Work out the finished part from the listing and answer in its coordinate system (mm). A direction names the side the tool comes from. Give positions to 0.01 mm unless a question says otherwise; leave off trailing zeros. Write each loop counter-clockwise with the first axis right and the second up, starting at its lowest first coordinate (ties: lowest second). Pieces come first, ordered by that corner, then holes. Notation, with made-up numbers: (-21, 62) - (-11, 62) arc R16 cw to (-11, 77) - close; hole circle Ø10 at (80, -23.5). An arc over 180 degrees is marked (long way). Write item = value, one per line.
from build123d import *

# Parameters (mm, degrees)
SKETCH3_R   = 12.7
SKETCH3_R_2 = 8.73125


with BuildPart() as part:
    # Sweep1: sweep along a path in Sketch1
    with BuildLine(Plane.XY) as sweep1_path:
        Line((0, 0), (0, 241.3))
        Line((0, 241.3), (736.6, 241.3))
        Line((736.6, 241.3), (736.6, 0))
    # Sketch3 → Sweep1 (sweep)
    with BuildSketch(Plane(origin=(0, 0, 0), x_dir=(1, 0, 0), z_dir=(0, 1, 0))):
        Circle(SKETCH3_R)
        Circle(SKETCH3_R_2, mode=Mode.SUBTRACT)
    sweep(path=sweep1_path.line, transition=Transition.RIGHT)


solid = part.part
1. Find section D-D, the plane y = 241.3. Give the vertices of the cut face in (x, z).
Solution:
outline = (0, -12.7) - (736.6, -12.7) arc R12.7 ccw to (736.6, 12.7) - (0, 12.7) arc R12.7 ccw to start; hole (0, -8.73) - (736.6, -8.73) arc R8.73 ccw to (736.6, 8.73) - (0, 8.73) arc R8.73 ccw to start
2. Given pin 1 (4 mm diameter, centred on y = 35.5, z = -4, fed in from +X); pin 2 (5 mm diameter, centred on y = 190.5, z = -9, fed in from +X); pin 3 (12 mm diameter, centred on y = 140, z = 8.5, fed in from -X), each flat-ended and moving along its own axis, determine where each tip first touches the part or whether it passes through.
Solution:
pin_1 = 749.14
pin_2 = 747.51
pin_3 = -12.45
3. Straight lines are drawn through the part: line 1 (X direction, y = 116.5, z = -0.5); line 2 (Z direction, x = 736.6, y = 65.5); line 3 (Y direction, x = 76.5, z = -1.5). For each, find the intervals that lie inside material, in ascending order.
Solution:
line_1 = -12.69 to -8.72, 8.72 to 12.69, 723.91 to 727.88, 745.32 to 749.29
line_2 = -12.7 to -8.73, 8.73 to 12.7
line_3 = 228.69 to 232.7, 249.9 to 253.91
4. Find section C-C, the plane y = 190.5. Give the vertices of the cut face in (x, z).
Solution:
outline = circle Ø25.4 at (0, 0); circle Ø25.4 at (736.6, 0); hole circle Ø17.46 at (0, 0); hole circle Ø17.46 at (736.6, 0)
5. A tool of negligible diameter and unlimited length cuts with its end or side. For faces 4 (the cylindrical face through (-12.688, 128.778, -0.558)), 5 (the flat face through (728, 0, 3)), from which of +Z, -Z, +X, -X, +Y, -Y can it reach the whole face along a straight path? Write none if from no direction.
Solution:
face_4 = -Y
face_5 = +Z, -Z, +X, -X, -Y
6. Find section B-B, the plane x = 736.6. Give the vertices of the cut face in (y, z).
Solution:
outline = (0, -12.7) - (241.3, -12.7) arc R12.7 ccw to (241.3, 12.7) - (0, 12.7) - (0, 8.73) - (241.3, 8.73) arc R8.73 cw to (241.3, -8.73) - (0, -8.73) - close
7. Find section A-A, the plane z = 0. Give the vertices of the cut face in (x, y), then the cut area to 3 significant figures.
Solution:
outline = (-12.7, 0) - (-8.73, 0) - (-8.73, 250.03) - (745.33, 250.03) - (745.33, 0) - (749.3, 0) - (749.3, 254) - (-12.7, 254) - close; (8.73, 0) - (12.7, 0) - (12.7, 228.6) - (723.9, 228.6) - (723.9, 0) - (727.87, 0) - (727.87, 232.57) - (8.73, 232.57) - close
area = 9,680 mm^2
8. For a pull along Z with two mould halves and no side action, classify faces 1 (the flat face through (9, 0, 3)), 2 (the cylindrical face through (373.634, 229.186, -3.815)), 3 (the cylindrical face through (373.578, 250.023, -0.384)) as pulls with the +Z half, pulls with the -Z half, needs draft (parallel to the pull), parting line crosses it, or undercut.
Solution:
face_1 = needs draft
face_2 = parting line crosses it
face_3 = undercut
